Autodesk Inventor part; units mm, degrees
ref_plane "YZ Plane" through (0, 0, 0) normal (1, 0, 0) x (0, 1, 0)
ref_plane "XZ Plane" through (0, 0, 0) normal (0, 1, 0) x (-1, 0, 0)
ref_plane "XY Plane" through (0, 0, 0) normal (0, 0, 1) x (1, 0, 0)
sketch "Sketch1" plane through (0, 0, 0) normal (0, 1, 0) x (-1, 0, 0)
  circle A0 centre (0, 0) radius 12.7
  dimension "d0" = 25.4
extrude "Extrusion1" add sketch "Sketch1" along normal blind 279.4
shell "Shell1" thickness 2.54 removed faces 1 at (3.6254, 279.4, -0.9542)
sketch "Sketch2" plane through (0, 0, 0) normal (0, -1, 0) x (1, 0, 0)
  line L0 (-12.7, 12.7) -> (12.7, 12.7)
  line L1 (12.7, 12.7) -> (12.7, -12.7)
  line L2 (12.7, -12.7) -> (-12.7, -12.7)
  line L3 (-12.7, -12.7) -> (-12.7, 12.7)
  point P0 (0, 0)
  point P1 (0, 0)
  dimension "d5" = 25.4
  dimension "d6" = 25.4
extrude "Extrusion2" add sketch "Sketch2" along normal blind 25.4
sketch "Sketch3" plane through (12.7, 0, -12.7) normal (0, 0, -1) x (-1, 0, 0)
  line L0 (0, 0) -> (0, -25.4)
  line L1 (25.4, 0) -> (25.4, -25.4)
  circle A0 centre (12.7, -12.7) radius 6.35
  point P0 (12.7, 0)
  dimension "d9" = 12.7
extrude "Extrusion3" cut sketch "Sketch3" against normal blind 33.3375
fillet "Fillet1" radius 12.7 2 edges at (12.7, -25.4, 0) (-12.7, -25.4, 0)
properties part number "ElevatorCylinderOuter"
Work out the finished part from the listing and answer in its coordinate system (mm). A direction names the side the tool comes from. Give positions to 0.01 mm unless a question says otherwise; leave off trailing zeros. Write each loop counter-clockwise with the first axis right and the second up, starting at its lowest first coordinate (ties: lowest second). Pieces come first, ordered by that corner, then holes. Notation, with made-up numbers: (44, -30.75) - (58, -30.75) arc R14 cw to (58, -19.75) - close; hole circle Ø8 at (30, 49.5). An arc over 180 degrees is marked (long way). One line per item, written item: value. Start each with the question number.
1. Find section B-B (y = 53). Write down the section's boundary in (x, z).
2. Consider probe 1 along Z at (x, y) = (0, 184); probe 2 along X at (y, z) = (140, 1); probe 3 along Z at (x, y) = (0.5, 212.5). Determine where each line is inside the solid, lowest interval first.
3. For a pull along X with two mould halves and no side action, classify faces 6 (the flat face through (6, 279.4, 9)), 7 (the flat face through (-12.7, -6, 0)), 8 (the cylindrical face through (1.38, -18.9, -0.18)), 9 (the flat face through (0, 2.54, 0)) as +X half, -X half, draft (parallel to the pull), parting line (faces both ways), or undercut.
4. For faces 1 (the flat face through (-10, 0, -10)), 2 (the flat face through (10, 0, 10)), 3 (the flat face through (10, 0, -10)), 4 (the flat face through (-10, 0, 10)), 5 (the cylindrical face through (1.323, 139.032, -10.074)), determine the directions among +Z, -Z, +X, -X, +Y, -Y from which every point of the face is accessible in a straight line to the end or side of a thin tool.
5. Given pin 1 (12 mm diameter, centred on y = 230.5, z = 6.5, fed in from -X); pin 2 (3 mm diameter, centred on x = 7, z = -5, fed in from +Y); pin 3 (2 mm diameter, centred on y = 221.5, z = 1.5, fed in from +X), each flat-ended and moving along its own axis, determine where each tip first touches the part or whether it passes through.
Geometry results:
1. outline: circle Ø25.4 at (0, 0); hole circle Ø20.32 at (0, 0)
2. probe 1: -12.7 to -10.16, 10.16 to 12.7
2. probe 2: -12.66 to -10.11, 10.11 to 12.66
2. probe 3: -12.69 to -10.15, 10.15 to 12.69
3. face 6: draft
3. face 7: -X half
3. face 8: undercut
3. face 9: undercut
4. face 1: -Z, -X, +Y
4. face 2: +Z, +X, +Y
4. face 3: -Z, +X, +Y
4. face 4: +Z, -X, +Y
4. face 5: +Y
5. pin 1: x = -12.69
5. pin 2: y = 2.54
5. pin 3: x = 12.69
